Could you check a few things on this model? Use its own coordinates, in mm. A direction names the side the tool comes from. Round coordinates to 2 decimals unless told otherwise and drop trailing zeros. Write each loop counter-clockwise with the first axis right and the second up, starting at its lowest first coordinate (ties: lowest second). Pieces come first, ordered by that corner, then holes. Notation, with made-up numbers: (61.25, 43.5) - (98.25, 43.5) arc R31 cw to (98.25, 74.5) - close; hole circle Ø7 at (87, 14). An arc over 180 degrees is marked (long way). Put each result on its own line as item: value.
from build123d import *

# Parameters (mm, degrees)
SKETCH1_R           = 3.645
BOSS_EXTRUDE1_DEPTH = 93.98
SKETCH2_R           = 4
CUT_EXTRUDE1_DEPTH  = 93.98


with BuildPart() as part:
    # Sketch1 → Boss-Extrude1 (new body)
    with BuildSketch(Plane(origin=(0, 0, 0), x_dir=(1, 0, 0), z_dir=(0, 1, 0))):
        with BuildLine():
            Line((11.476895811, 1.535297401), (16.201895811, 1.535297401))
            Line((16.201895811, 1.535297401), (10.051895811, 7.685297401))
            Line((10.051895811, 7.685297401), (2.051895811, 7.685297401))
            Line((2.051895811, 7.685297401), (-4.098104189, 1.535297401))
            Line((-4.098104189, 1.535297401), (0.626895811, 1.535297401))
            ThreePointArc((0.626895811, 1.535297401), (2.051895811, 0.110297401), (0.626895811, -1.314702599))
            Line((0.626895811, -1.314702599), (-7.549539962, -1.288266826))
            ThreePointArc((-7.549539962, -1.288266826), (-8.538474211, -0.878636848), (-8.948104189, 0.110297401))
            Line((-8.948104189, 0.110297401), (-8.948104189, 8.260297401))
            ThreePointArc((-8.948104189, 8.260297401), (-7.549539962, 9.658861629), (-6.150975734, 8.260297401))
            Line((-6.150975734, 8.260297401), (-6.150975734, 3.535297401))
            Line((-6.150975734, 3.535297401), (-0.000975734, 9.685297401))
            Line((-0.000975734, 9.685297401), (-0.000975734, 17.685297401))
            Line((-0.000975734, 17.685297401), (-6.150975734, 23.835297401))
            Line((-6.150975734, 23.835297401), (-6.150975734, 19.110297401))
            ThreePointArc((-6.150975734, 19.110297401), (-7.575975734, 17.685297401), (-9.000975734, 19.110297401))
            Line((-9.000975734, 19.110297401), (-9.000975734, 27.260250811))
            ThreePointArc((-9.000975734, 27.260250811), (-8.583602897, 28.267877974), (-7.575975734, 28.685250811))
            Line((-7.575975734, 28.685250811), (0.574024266, 28.685250811))
            ThreePointArc((0.574024266, 28.685250811), (1.999024266, 27.260250811), (0.574024266, 25.835250811))
            Line((0.574024266, 25.835250811), (-4.150975734, 25.835250811))
            Line((-4.150975734, 25.835250811), (1.999024266, 19.685250811))
            Line((1.999024266, 19.685250811), (9.999024266, 19.685250811))
            Line((9.999024266, 19.685250811), (16.149024266, 25.835250811))
            Line((16.149024266, 25.835250811), (11.424024266, 25.835250811))
            ThreePointArc((11.424024266, 25.835250811), (9.999024266, 27.260250811), (11.424024266, 28.685250811))
            Line((11.424024266, 28.685250811), (19.574024266, 28.685250811))
            ThreePointArc((19.574024266, 28.685250811), (20.581651429, 28.267877974), (20.999024266, 27.260250811))
            Line((20.999024266, 27.260250811), (20.999024266, 19.213994497))
            ThreePointArc((20.999024266, 19.213994497), (19.574024266, 17.788994497), (18.149024266, 19.213994497))
            Line((18.149024266, 19.213994497), (18.149024266, 23.835250811))
            Line((18.149024266, 23.835250811), (11.999024266, 17.685250811))
            Line((11.999024266, 17.685250811), (11.999024266, 9.685250811))
            Line((11.999024266, 9.685250811), (18.149024266, 3.535250811))
            Line((18.149024266, 3.535250811), (18.149024266, 8.363994497))
            ThreePointArc((18.149024266, 8.363994497), (19.574024266, 9.788994497), (20.999024266, 8.363994497))
            Line((20.999024266, 8.363994497), (20.999024266, 0.110297401))
            ThreePointArc((20.999024266, 0.110297401), (20.581651429, -0.897329762), (19.574024266, -1.314702599))
            Line((19.574024266, -1.314702599), (11.476895811, -1.314702599))
            ThreePointArc((11.476895811, -1.314702599), (10.051895811, 0.110297401), (11.476895811, 1.535297401))
        make_face()
        with Locations(Location((6.051895811, 13.685297401, 0), (0, 0, 270))):
            Circle(SKETCH1_R, mode=Mode.SUBTRACT)
    extrude(amount=BOSS_EXTRUDE1_DEPTH)

    # Sketch2 → Cut-Extrude1 (cut)
    with BuildSketch(Plane(origin=(11.999024266, 0, 0), x_dir=(0, 0, -1), z_dir=(1, 0, 0))):
        with Locations((13.685250811, 75.14)):
            Circle(SKETCH2_R)
        with Locations((13.685250811, 18.84)):
            Circle(SKETCH2_R)
    extrude(amount=-CUT_EXTRUDE1_DEPTH, mode=Mode.SUBTRACT)


solid = part.part
(1) For faces 1 (the face through (3, 93.98, -17)), 2 (the face through (2, 46.3, -27.3)), which set-ups out of +Z, -Z, +X, -X, +Y, -Y let a thin tool reach every point of the face, with its end or its side?
Values found:
face 1: +Z, -Z, +X, -X, +Y
face 2: +Y, -Y
(2) Imagine slicing it at C-C, the plane z = -5.5. List the corners of the cut face in (x, y) for me, then the cut area to 3 significant figures.
Values found:
outline: (-8.95, 0) - (-6.15, 0) - (-6.15, 93.98) - (-8.95, 93.98) - close; (-4.19, 0) - (-0.13, 0) - (-0.13, 93.98) - (-4.19, 93.98) - close; (12.24, 0) - (16.18, 0) - (16.18, 93.98) - (12.24, 93.98) - close; (18.15, 0) - (21, 0) - (21, 93.98) - (18.15, 93.98) - close
area: 1,280 mm^2
(3) I'm going to push flat-ended pins straight in: pin 1 (9 mm diameter, centred on y = 84.5, z = -13.5, fed in from +X); pin 2 (6.5 mm diameter, centred on x = 6.05, z = -13.69, fed in from -Y); pin 3 (10.5 mm diameter, centred on y = 18.84, z = -13.69, fed in from +X); pin 4 (4 mm diameter, centred on x = 5, y = 35, fed in from -Z). Where does each tip first touch, or does it pass through?
Values found:
pin 1: stops at x = 20.85
pin 2: passes through
pin 3: stops at x = 21
pin 4: stops at z = -19.69
(4) Imagine slicing it at B-B, the plane z = -13.75. List the corners of the cut face in (x, y) for me, then the cut area to 3 significant figures.
Values found:
outline: (0, 0) - (2.41, 0) - (2.41, 14.84) - (0, 14.84) - close; (0, 22.84) - (2.41, 22.84) - (2.41, 71.14) - (0, 71.14) - close; (0, 79.14) - (2.41, 79.14) - (2.41, 93.98) - (0, 93.98) - close; (9.7, 0) - (12, 0) - (12, 14.84) - (9.7, 14.84) - close; (9.7, 22.84) - (12, 22.84) - (12, 71.14) - (9.7, 71.14) - close; (9.7, 79.14) - (12, 79.14) - (12, 93.98) - (9.7, 93.98) - close
area: 367 mm^2
(5) If we mould it in two halves opening along Z, with no side actions, what happens to faces 3 (the face through (20.999, 46, -4)), 4 (the face through (6, 46, -19.685)), 5 (the face through (18.149, 46, -6))? For each: pulls with the +Z half, pulls with the -Z half, needs draft (parallel to the pull), parting line crosses it, or undercut.
Values found:
face 3: needs draft
face 4: pulls with the -Z half
face 5: undercut
(6) Imagine slicing it at A-A, the plane x = -1. List the corners of the cut face in (y, z) for me, then the cut area to 3 significant figures.
Values found:
outline: (0, -28.69) - (93.98, -28.69) - (93.98, -25.84) - (0, -25.84) - close; (0, -22.68) - (93.98, -22.68) - (93.98, -18.68) - (0, -18.68) - close; (0, -8.69) - (93.98, -8.69) - (93.98, -4.63) - (0, -4.63) - close; (0, -1.54) - (93.98, -1.54) - (93.98, 1.31) - (0, 1.31) - close
area: 1,290 mm^2
(7) Please list where these lines run through material, in increasing order: probe 1 along X at (y, z) = (73.5, -23.5); probe 2 along X at (y, z) = (7, -20.5); probe 3 along Z at (x, y) = (9, 75). Write a range as from..to.
Values found:
probe 1: x = -9..-6.15, -5.82..-1.82, 13.81..17.81, 18.15..21
probe 2: x = -9..-6.15, -2.82..1.18, 10.81..14.81, 18.15..21
probe 3: z = -19.69..-17.68, -9.69..-7.69
